Geometry check sheet. Reference: the model listing, model coordinates, mm. A direction names the side the tool comes from. Coordinates: 2 decimals unless noted, no trailing zeros. Loops run counter-clockwise (first coordinate to the right, second up) from the corner with the lowest first, then second, coordinate; pieces in that order, holes last. Notation, with made-up numbers: (77.5, 86) - (119.5, 86) arc R10 cw to (119.5, 105) - close; hole circle Ø7 at (-12, 57). An arc over 180 degrees is marked (long way). One line per item, written item: value.
Autodesk Inventor part; units mm, degrees
ref_plane "YZ Plane" through (0, 0, 0) normal (1, 0, 0) x (0, 1, 0)
ref_plane "XZ Plane" through (0, 0, 0) normal (0, 1, 0) x (-1, 0, 0)
ref_plane "XY Plane" through (0, 0, 0) normal (0, 0, 1) x (1, 0, 0)
sketch "Sketch1" plane through (0, 0, 0) normal (0, 1, 0) x (-1, 0, 0)
  line L0 (0, 0) -> (25.4, 0)
  line L1 (25.4, 0) -> (25.4, -3.175)
  line L2 (25.4, -3.175) -> (0, -3.175)
  line L3 (0, -3.175) -> (0, 0)
  line L4 (0, 0) -> (3.175, 0)
  line L5 (3.175, 0) -> (3.175, -25.4)
  line L6 (3.175, -25.4) -> (0, -25.4)
  line L7 (0, -25.4) -> (0, 0)
  dimension "d0" = 25.4
  dimension "d1" = 3.175
  dimension "d2" = 3.175
  dimension "d3" = 25.4
extrude "Extrusion1" add sketch "Sketch1" along normal blind 76.2
sketch "Sketch2" plane through (0, 0, 0) normal (1, 0, 0) x (0, 0, -1)
  line L0 (0, 0) -> (25.4, 0)
  line L1 (25.4, 0) -> (25.4, 76.2)
  point P0 (19.05, 6.35)
  point P1 (6.35, 19.05)
  dimension "d6" = 6.35
  dimension "d7" = 6.35
  dimension "d8" = 19.05
  dimension "d9" = 19.05
hole "Hole1" at (0, 6.35, -19.05) at (0, 19.05, -6.35) direction (-1, 0, 0) diameter 6.35 end through all
properties part number "1x1 angle mechanical stop"
(1) Cross-section at C-C on y = 53. Record the cut outline in (x, z) (3 decimals).
Reply:
outline: (-25.4, -3.175) - (-3.175, -3.175) - (-3.175, -25.4) - (0, -25.4) - (0, 0) - (-25.4, 0) - close
(2) Material ranges on probe 1 along Z at (x, y) = (-1.9, 19.05) (3 decimals); probe 2 along Y at (x, z) = (-1.7, -19.05) (3 decimals); probe 3 along Y at (x, z) = (-1.15, -6.35) (3 decimals), recorded low to high. Write a range as from..to.
Reply:
probe 1: -25.4..-9.525, -3.175..0
probe 2: 0..3.175, 9.525..76.2
probe 3: 0..15.875, 22.225..76.2
(3) Cross-section at D-D on x = -8.5. Record the cut outline in (y, z) (3 decimals).
Reply:
outline: (0, -3.175) - (76.2, -3.175) - (76.2, 0) - (0, 0) - close
(4) Release check for a two-part mould opening along Y. For faces 3 (the face through (-2, 0, -7)), 4 (the face through (-1.61, 6.21, -15.88)), 5 (the face through (0, 38, -13)) record: pulls with the +Y half, pulls with the -Y half, needs draft (parallel to the pull), parting line crosses it, or undercut.
Reply:
face 3: pulls with the -Y half
face 4: undercut
face 5: needs draft
(5) Cross-section at B-B on y = 6.35. Record the cut outline in (x, z) (3 decimals), and give its area (3 significant figures).
Reply:
outline: (-25.4, -3.175) - (-3.175, -3.175) - (-3.175, -15.875) - (0, -15.875) - (0, 0) - (-25.4, 0) - close; (-3.175, -25.4) - (0, -25.4) - (0, -22.225) - (-3.175, -22.225) - close
area: 131 mm2
(6) Go/stop test with flat-tipped pins: pin 1 Ø10 at (x, y) = (-3.5, 18) entering from +Z; pin 2 Ø7.5 at (y, z) = (6.35, -19.05) entering from -X (3 decimals); pin 3 Ø4 at (x, y) = (-14, 23.5) entering from -Z (3 decimals). Record where each tip stops, or that it passes through.
Reply:
pin 1: z = 0
pin 2: x = -3.175
pin 3: z = -3.175
(7) Cross-section at A-A on z = -6.35. Record the cut outline in (x, y) (3 decimals), and give its area (3 significant figures).
Reply:
outline: (-3.175, 0) - (0, 0) - (0, 15.875) - (-3.175, 15.875) - close; (-3.175, 22.225) - (0, 22.225) - (0, 76.2) - (-3.175, 76.2) - close
area: 222 mm2
(8) Access from +Z, -Z, +X, -X, +Y, -Y to the whole of each face (thin tool, end or side, straight path). Record for faces 1 (the face through (-2, 38, -25.4)), 2 (the face through (-14, 38, -3.175)).
Reply:
face 1: -Z, +X, -X, +Y, -Y
face 2: -Z, -X, +Y, -Y
